from build123d import *

# Parameters (mm, degrees)
SKETCH1_R           = 22.987
BOSS_EXTRUDE1_DEPTH = 16.764
SKETCH2_R           = 20.828
BOSS_EXTRUDE2_DEPTH = 24.384
SKETCH3_R           = 7.366
BOSS_EXTRUDE3_DEPTH = 4.318
BOSS_EXTRUDE4_START = 6.858
SKETCH4_R           = 20.828
BOSS_EXTRUDE4_DEPTH = 6.858
SKETCH5_R           = 7.239
BOSS_EXTRUDE5_DEPTH = 4.572
SKETCH6_R           = 2.413
BOSS_EXTRUDE6_DEPTH = 13.97
SKETCH7_R           = 4.572
BOSS_EXTRUDE7_DEPTH = 9.144
SKETCH8_RX          = 1.524
SKETCH8_RY          = 0.508
BOSS_EXTRUDE8_DEPTH = 9.144
CIRPATTERN1_COUNT   = 15


with BuildPart() as part:
    # Sketch1 → Boss-Extrude1 (new, symmetric)
    with BuildSketch(Plane.XY):
        Circle(SKETCH1_R)
    extrude(amount=BOSS_EXTRUDE1_DEPTH, both=True)

    # Sketch2 → Boss-Extrude2 (add)
    with BuildSketch(Plane(origin=(0, 0, -16.764), x_dir=(-1, 0, 0), z_dir=(0, 0, -1))):
        with Locations(Location((0, 0, 0), (0, 0, 180))):
            Circle(SKETCH2_R)
    extrude(amount=BOSS_EXTRUDE2_DEPTH)

    # Sketch3 → Boss-Extrude3 (add)
    with BuildSketch(Plane(origin=(0, 0, -41.148), x_dir=(-1, 0, 0), z_dir=(0, 0, -1))):
        Circle(SKETCH3_R)
    extrude(amount=BOSS_EXTRUDE3_DEPTH)

    # Sketch4 → Boss-Extrude4 (add)
    with BuildSketch(Plane.XY.offset(16.764).offset(BOSS_EXTRUDE4_START)):
        Circle(SKETCH4_R)
    extrude(amount=-BOSS_EXTRUDE4_DEPTH)

    # Sketch5 → Boss-Extrude5 (add)
    with BuildSketch(Plane.XY.offset(23.622)):
        Circle(SKETCH5_R)
    extrude(amount=BOSS_EXTRUDE5_DEPTH)

    # Sketch6 → Boss-Extrude6 (add)
    with BuildSketch(Plane.XY.offset(28.194)):
        Circle(SKETCH6_R)
    extrude(amount=BOSS_EXTRUDE6_DEPTH)

    # Sketch7 → Boss-Extrude7 (add)
    with BuildSketch(Plane.XY.offset(28.194)):
        with Locations(Location((0, 0, 0), (0, 0, 180))):
            Circle(SKETCH7_R)
    extrude(amount=BOSS_EXTRUDE7_DEPTH)

    # Sketch8 → Boss-Extrude8 (add)
    with BuildSketch(Plane.XY.offset(28.194)):
        with Locations(Location((0, 4.572), (0, 0, 90))):
            Ellipse(SKETCH8_RX, SKETCH8_RY)
    boss_extrude8 = extrude(amount=BOSS_EXTRUDE8_DEPTH)

    # CirPattern1: Boss-Extrude8 ×15 about axis
    cirpattern1_axis = Axis((0, 0, -49.8475), (0, 0, 1))
    for i in range(1, CIRPATTERN1_COUNT):
        add(boss_extrude8.rotate(cirpattern1_axis, i * 360 / CIRPATTERN1_COUNT))


solid = part.part
Could you check a few things on this model? Use its own coordinates, in mm. A direction names the side the tool comes from. Give positions to 0.01 mm unless a question says otherwise; leave off trailing zeros. Order: outer loops, then holes, each group sorted by start corner. A loop starts at its lowest first (then second) coordinate and runs counter-clockwise, first axis right, second up.
Item 1: For faces 1 (the face through (9, 0, 23.622)), 2 (the face through (0, 0, -45.466)), 3 (the face through (-3.399, -6.535, -43.277)), which set-ups out of +Z, -Z, +X, -X, +Y, -Y let a thin tool reach every point of the face, with its end or its side?
Item 2: If we section it at C-C, the plane z = 9: Write out the boundary of the cut face in (x, y).
Item 3: I'm going to push flat-ended pins straight in: pin 1 (4 mm diameter, centred on y = 17.5, z = -5.5, fed in from +X); pin 2 (3 mm diameter, centred on x = -14, z = -15, fed in from +Y); pin 3 (4 mm diameter, centred on x = -3, y = 13, fed in from -Z). Where does each tip first touch, or does it pass through?
Item 4: I need wall thicknesses on line 1 (Z direction, x = -13.5, y = -16); line 2 (Z direction, x = -2.5, y = -4); line 3 (X direction, y = -10.5, z = -1.5). Which ranges of each line are inside material? Lowest first, please.
Item 5: If we section it at A-A, the plane x = 13: Write out the boundary of the cut face in (y, z).
Item 6: If we section it at B-B, the plane z = -23.5: Write out the boundary of the cut face in (x, y), plus the area to 3 significant figures.
Values:
1. face 1: +Z
1. face 2: -Z, +X, -X, +Y, -Y
1. face 3: -Z
2. outline: circle Ø45.97 at (0, 0)
3. pin 1: stops at x = 16.98
3. pin 2: stops at y = 19.29
3. pin 3: stops at z = -41.15
4. line 1: z = -16.76 to 16.76
4. line 2: z = -45.47 to 37.34
4. line 3: x = -20.45 to 20.45
5. outline: (-18.96, -16.76) - (-16.27, -16.76) - (-16.27, -41.15) - (16.27, -41.15) - (16.27, -16.76) - (18.96, -16.76) - (18.96, 16.76) - (16.27, 16.76) - (16.27, 23.62) - (-16.27, 23.62) - (-16.27, 16.76) - (-18.96, 16.76) - close
6. outline: circle Ø41.66 at (0, 0)
6. area: 1,360 mm2
